Could you check a few things on this model? Use its own coordinates, in mm. A direction names the side the tool comes from. Give positions to 0.01 mm unless a question says otherwise; leave off trailing zeros. Write each loop counter-clockwise with the first axis right and the second up, starting at its lowest first coordinate (ties: lowest second). Pieces come first, ordered by that corner, then holes. Notation, with made-up numbers: (60.25, 48) - (90.25, 48) arc R9 cw to (90.25, 60) - close; hole circle Ø5 at (56.25, -20.75). An arc over 180 degrees is marked (long way). Answer as a JSON object with one key per item and string values. Group by question number.
```python
from build123d import *


with BuildPart() as f1:
    # F0 (on Front) → F1 (revolve)
    with BuildSketch(Plane.XZ):
        with BuildLine():
            Line((-3, 32), (-3, 30))
            Line((-3, 30), (0, 30))
            Line((0, 30), (3, 30))
            Line((3, 30), (3, 32))
            Line((3, 32), (18, 32))
            Line((18, 32), (18, 33))
            Line((18, 33), (21, 33))
            Line((21, 33), (21, 32))
            Line((21, 32), (24, 32))
            Line((24, 32), (24, 40.5))
            Line((24, 40.5), (14, 40.5))
            ThreePointArc((14, 40.5), (12.585786, 41.085786), (12, 42.5))
            Line((12, 42.5), (12, 62))
            ThreePointArc((12, 62), (12.585786, 63.414214), (14, 64))
            Line((14, 64), (24, 64))
            Line((24, 64), (24, 80.5))
            Line((24, 80.5), (0, 80.5))
            Line((0, 80.5), (-24, 80.5))
            Line((-24, 80.5), (-24, 64))
            Line((-24, 64), (-14, 64))
            ThreePointArc((-14, 64), (-12.585786, 63.414214), (-12, 62))
            Line((-12, 62), (-12, 42.5))
            ThreePointArc((-12, 42.5), (-12.585786, 41.085786), (-14, 40.5))
            Line((-14, 40.5), (-24, 40.5))
            Line((-24, 40.5), (-24, 32))
            Line((-24, 32), (-21, 32))
            Line((-21, 32), (-21, 33))
            Line((-21, 33), (-18, 33))
            Line((-18, 33), (-18, 32))
            Line((-18, 32), (-3, 32))
        make_face()
    revolve(axis=Axis((10.5, 0, 32), (1, 0, 0)))


solid = f1.part
```
(1) Will these pins go through, and if not, where does the flat tip stop? P1, Ø1.5, axis at x = -5, y = 38.5, coming from the +Z side; P2, Ø12, axis at x = 18, y = 28.5, coming from the -Z side; P3, Ø5, axis at x = 6, y = 17.5, coming from the -Z side.
(2) I want a section at B-B, the plane x = -9. Please give me the cut outline in (y, z).
(3) I want a section at A-A, the plane y = 36. Please give me the cut outline in (x, z), and give its area (3 significant figures).
(4) I need wall thicknesses on L1, parallel to Y at x = -19, z = 32; L2, parallel to Z at x = -20, y = 0; L3, parallel to Z at x = 17, y = 0. Which ranges of each line are inside material? Lowest first, please.
(5) If we mould it in two halves opening along Z, with no side actions, what happens to faces 1 (the cylindrical face through (-0.34, 29.51, -6.49)), 2 (the flat face through (-24, 0, 32)), 3 (the cylindrical face through (19.07, 31.24, 25.06))? For each: +Z half, -Z half, draft (parallel to the pull), parting line (faces both ways), or undercut.
(6) For faces 4 (the cylindrical face through (-19.07, -7.167, 36.57)), 5 (the flat face through (24, 10, 0)), 6 (the flat face through (12, 13, 32)), 7 (the cylindrical face through (0.042, 0.601, 30.092)), which set-ups out of +Z, -Z, +X, -X, +Y, -Y let a thin tool reach every point of the face, with its end or its side?
Entries:
{
 "1": {"P1": "z = 62.45", "P2": "z = -10.97", "P3": "z = -14.12"},
 "2": {"outline": "circle Ø97 at (0, 32)"},
 "3": {"outline": "(-24, -0.5) - (24, -0.5) - (24, 64.5) - (-24, 64.5) - close", "area": "3,120 mm^2"},
 "4": {"L1": "-48.5 to -32, -8.5 to -1, 1 to 8.5, 32 to 48.5", "L2": "-16.5 to 0, 23.5 to 31, 33 to 40.5, 64 to 80.5", "L3": "-16.5 to 0, 23.5 to 40.5, 64 to 80.5"},
 "5": {"face 1": "parting line", "face 2": "draft", "face 3": "undercut"},
 "6": {"face 4": "-X", "face 5": "+Z, -Z, +X, +Y, -Y", "face 6": "+X", "face 7": "none"}
}
